from build123d import *

# Parameters (mm, degrees)
BOSS_EXTRUDE2_DEPTH      = 5.08
FILLET1_R                = 2.032
CUT_EXTRUDE1_DEPTH       = 24.94682426
BOSS_EXTRUDE3_DEPTH      = 4.143000096
BOSS_EXTRUDE3_DEPTH_BACK = 7.62
SKETCH7_R                = 9.525


with BuildPart() as part:
    # Sketch5 → Boss-Extrude2 (new body)
    with BuildSketch(Plane.XY):
        with BuildLine():
            ThreePointArc((13.895294195, 3.040226179), (15.067976, 8.6995), (9.580560202, 10.513564677))
            ThreePointArc((9.580560202, 10.513564677), (7.112, 12.318345343), (4.314733993, 13.553790856))
            ThreePointArc((4.314733993, 13.553790856), (0, 17.399), (-4.314733993, 13.553790856))
            ThreePointArc((-4.314733993, 13.553790856), (-7.112, 12.318345343), (-9.580560202, 10.513564677))
            ThreePointArc((-9.580560202, 10.513564677), (-15.067976, 8.6995), (-13.895294195, 3.040226179))
            ThreePointArc((-13.895294195, 3.040226179), (-14.224, 0), (-13.895294195, -3.040226179))
            ThreePointArc((-13.895294195, -3.040226179), (-15.067976, -8.6995), (-9.580560202, -10.513564677))
            ThreePointArc((-9.580560202, -10.513564677), (-7.112, -12.318345343), (-4.314733993, -13.553790856))
            ThreePointArc((-4.314733993, -13.553790856), (0, -17.399), (4.314733993, -13.553790856))
            ThreePointArc((4.314733993, -13.553790856), (7.112, -12.318345343), (9.580560202, -10.513564677))
            ThreePointArc((9.580560202, -10.513564677), (15.067976, -8.6995), (13.895294195, -3.040226179))
            ThreePointArc((13.895294195, -3.040226179), (14.224, 0), (13.895294195, 3.040226179))
        make_face()
    extrude(amount=BOSS_EXTRUDE2_DEPTH)

    # Fillet1
    fillet1_edges = [part.edges().sort_by_distance(p)[0] for p in [
        (-4.314733993, 13.553790856, 2.54),
        (4.314733993, 13.553790856, 2.54),
        (9.580560202, 10.513564677, 2.54),
        (13.895294195, 3.040226179, 2.54),
        (13.895294195, -3.040226179, 2.54),
        (9.580560202, -10.513564677, 2.54),
        (4.314733993, -13.553790856, 2.54),
        (-4.314733993, -13.553790856, 2.54),
        (-9.580560202, -10.513564677, 2.54),
        (-13.895294195, -3.040226179, 2.54),
        (-9.580560202, 10.513564677, 2.54),
        (-13.895294195, 3.040226179, 2.54),
    ]]
    fillet(fillet1_edges, radius=FILLET1_R)

    # Sketch6 → Cut-Extrude1 (cut, through all)
    with BuildSketch(Plane.XY.offset(5.08)):
        Polygon((7.405671903, 0), (3.702835951, 6.4135), (-3.702835951, 6.4135), (-7.405671903, 0), (-3.702835951, -6.4135), (3.702835951, -6.4135), align=None)
    extrude(amount=-CUT_EXTRUDE1_DEPTH, mode=Mode.SUBTRACT)

    # Sketch7 → Boss-Extrude3 (add, two sides: drawn at the far end of the back side and taken through both)
    with BuildSketch(Plane(origin=(0, 0, 0), x_dir=(-1, 0, 0), z_dir=(0, 0, -1)).offset(-BOSS_EXTRUDE3_DEPTH_BACK)):
        Circle(SKETCH7_R)
        Polygon((-7.405671903, 0), (-3.702835951, 6.4135), (3.702835951, 6.4135), (7.405671903, 0), (3.702835951, -6.4135), (-3.702835951, -6.4135), align=None, mode=Mode.SUBTRACT)
    extrude(amount=BOSS_EXTRUDE3_DEPTH + BOSS_EXTRUDE3_DEPTH_BACK)


solid = part.part
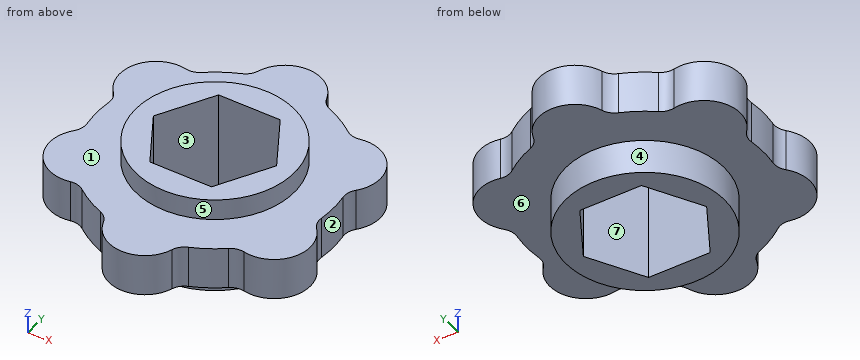
Part model, mm, in its own coordinate system. Face numbers are marked on the shaded views. A direction names the side the tool comes from. Give positions to 0.01 mm unless a question says otherwise; leave off trailing zeros. Write each loop counter-clockwise with the first axis right and the second up, starting at its lowest first coordinate (ties: lowest second). Pieces come first, ordered by that corner, then holes.
1) Cut at A-A on x = 0. Write the cut outline in (y, z) (1 decimal), then the cut area to 3 significant figures.
Resolved:
outline: (-17.4, 0) - (-9.5, 0) - (-9.5, -4.1) - (-6.4, -4.1) - (-6.4, 7.6) - (-9.5, 7.6) - (-9.5, 5.1) - (-17.4, 5.1) - close; (6.4, -4.1) - (9.5, -4.1) - (9.5, 0) - (17.4, 0) - (17.4, 5.1) - (9.5, 5.1) - (9.5, 7.6) - (6.4, 7.6) - close
area: 153 mm2
2) Probe L1, parallel to Y at x = 0, z = -2 (1 decimal); L2, parallel to Z at x = -3, y = -13.5; L3, parallel to Y at x = -2, z = 1. List the from-to ranges inside material, lowest first.
Resolved:
L1: y = -9.5 to -6.4, 6.4 to 9.5
L2: z = 0 to 5.08
L3: y = -16.91 to -6.41, 6.41 to 16.91
3) Which spindle directions (+Z, -Z, +X, -X, +Y, -Y) get a long thin tool onto all of the face, cutting with end or side? Do the marked faces 5, 6 and 7. Say none if no direction does.
Resolved:
face 5: +Z
face 6: -Z
face 7: +Z, -Z
4) Cut at C-C on y = -0.5. Write the cut outline in (x, z).
Resolved:
outline: (-14.22, 0) - (-9.51, 0) - (-9.51, -4.14) - (-7.12, -4.14) - (-7.12, 7.62) - (-9.51, 7.62) - (-9.51, 5.08) - (-14.22, 5.08) - close; (7.12, -4.14) - (9.51, -4.14) - (9.51, 0) - (14.22, 0) - (14.22, 5.08) - (9.51, 5.08) - (9.51, 7.62) - (7.12, 7.62) - close
5) Two-plate mould, pull along X, no slides. Class the marked faces 1, 2, 3 and 4: released by +X, released by -X, zero draft, split by the parting line, or undercut.
Resolved:
face 1: zero draft
face 2: released by +X
face 3: undercut
face 4: split by the parting line
6) Pin check, flat tips, straight feed: pin 1 (5 mm diameter, centred on x = 7, z = 0.5, fed in from +Y); pin 2 (6 mm diameter, centred on y = 9.5, z = 6, fed in from +X); pin 3 (6 mm diameter, centred on y = 12.5, z = 6, fed in from +X). Stop position of each tip, or through.
Resolved:
pin 1: stops at y = 13.77
pin 2: stops at x = 15.65
pin 3: stops at x = 14.33
7) Cut at D-D on y = -7.5. Write the cut outline in (x, z).
Resolved:
outline: (-15.54, 0) - (-5.87, 0) - (-5.87, -4.14) - (5.87, -4.14) - (5.87, 0) - (15.54, 0) - (15.54, 5.08) - (5.87, 5.08) - (5.87, 7.62) - (-5.87, 7.62) - (-5.87, 5.08) - (-15.54, 5.08) - close
